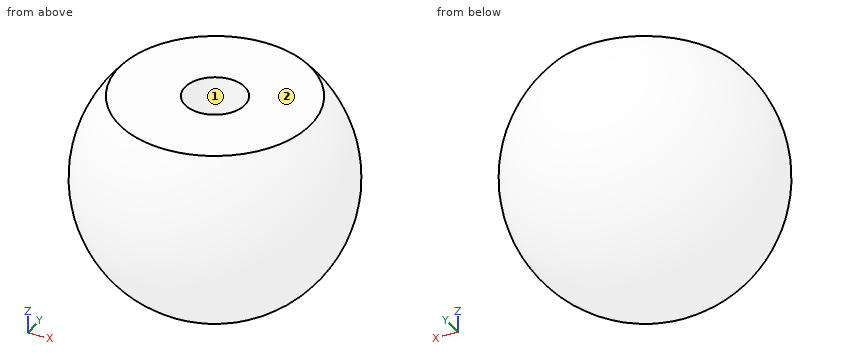
from build123d import *

# Parameters (mm, degrees)
CUT_EXTRUDE_1_DEPTH      = 16.588457268
CUT_EXTRUDE_1_DEPTH_BACK = 16.588457268
SKETCH_2_W               = 8.784286405
SKETCH_2_H               = 20.773221584
HOLE_WIZARD_M5_1_D       = 4.2
HOLE_WIZARD_M5_1_DEPTH   = 7
HOLE_WIZARD_M5_1_TIP     = 1.2618073


with BuildPart() as part:
    # 草图1 → 旋转1 (revolve)
    with BuildSketch(Plane(origin=(0, 0, 0), x_dir=(0, 0, -1), z_dir=(1, 0, 0))):
        with BuildLine():
            Line((0, 9), (0, -9))
            ThreePointArc((0, -9), (-9, 0), (0, 9))
        make_face()
    revolve(axis=Axis((0, 9, 0), (0, -1, 0)))

    # 草图2 → 切除-拉伸1 (cut, two sides: drawn at the far end of the back side and taken through both)
    with BuildSketch(Plane(origin=(0, 0, 0), x_dir=(0, 0, -1), z_dir=(1, 0, 0)).offset(-CUT_EXTRUDE_1_DEPTH_BACK)):
        with Locations((-10.392143203, 0)):
            Rectangle(SKETCH_2_W, SKETCH_2_H)
    extrude(amount=CUT_EXTRUDE_1_DEPTH + CUT_EXTRUDE_1_DEPTH_BACK, mode=Mode.SUBTRACT)

    # M5 螺纹孔1
    with Locations(Plane(origin=(0, 0, 6), x_dir=(0, 1, 0), z_dir=(0, 0, 1))):
        with Locations((0, 0)):
            Hole(HOLE_WIZARD_M5_1_D / 2, depth=HOLE_WIZARD_M5_1_DEPTH)
            with Locations((0, 0, -(HOLE_WIZARD_M5_1_DEPTH + HOLE_WIZARD_M5_1_TIP / 2))):  # 118° drill point
                Cone(0, HOLE_WIZARD_M5_1_D / 2, HOLE_WIZARD_M5_1_TIP, mode=Mode.SUBTRACT)


solid = part.part
Check sheet for the modelled part. Datum: model origin and axes. Units: mm. Face numbers are marked on the shaded views. Round coordinates to 2 decimals unless told otherwise and drop trailing zeros. Loops run counter-clockwise (first coordinate to the right, second up) from the corner with the lowest first, then second, coordinate; pieces in that order, holes last. Notation, with made-up numbers: M 12,84 L 21,84 A11 ccw 21,96 Z; hole C -34,37 d7. An arc over 180 degrees is marked long. One line per item, written item: value.
(1) Depth check by flat-ended pin: pin 1 Ø3 at (y, z) = (6, -2) entering from +X; pin 2 Ø6 at (x, y) = (6, 4.5) entering from -Z; pin 3 Ø2 at (x, z) = (-1.5, -3) entering from +Y. Enter the tip coordinate at first touch or a pass-through.
Computed values:
pin 1: stops at x = 7.6
pin 2: stops at z = -7.79
pin 3: stops at y = 8.69
(2) Sectioned sample at D-D, the plane z = -6.5. Record the cut outline in (x, y), then the cut area to 3 significant figures.
Computed values:
outline: C 0,0 d12.45
area: 122 mm^2
(3) Release check for a two-part mould opening along X. For the marked faces 1 and 2 record: +X half, -X half, draft (parallel to the pull), parting line (faces both ways), or undercut.
Computed values:
face 1: undercut
face 2: draft
(4) Sectioned sample at B-B, the plane z = 1.25. Record the cut outline in (x, y).
Computed values:
outline: C 0,0 d17.83; hole C 0,0 d4.2
(5) Sectioned sample at A-A, the plane x = -3. Record the cut outline in (y, z).
Computed values:
outline: M -6,6 A8.49 ccw long 6,6 Z
(6) Thickness scan on line 1 (X direction, y = 0, z = 3.5); line 2 (Y direction, x = -0.25, z = 1); line 3 (X direction, y = 0, z = 2.5). Record the ranges inside material, lowest first.
Computed values:
line 1: x = -8.29 to -2.1, 2.1 to 8.29
line 2: y = -8.94 to -2.09, 2.09 to 8.94
line 3: x = -8.65 to -2.1, 2.1 to 8.65
(7) Sectioned sample at C-C, the plane y = 7.25. Record the cut outline in (x, z).
Computed values:
outline: C 0,0 d10.67
